Design review of the part built by this model. Coordinates are the model's own, in mm. A direction names the side the tool comes from. Coordinates: 2 decimals unless noted, no trailing zeros. Write each loop counter-clockwise with the first axis right and the second up, starting at its lowest first coordinate (ties: lowest second). Pieces come first, ordered by that corner, then holes. Notation, with made-up numbers: M -1.5,-11.75 L 31.5,-11.75 A20 cw 31.5,13.25 Z; hole C 12.5,-20 d8. An arc over 180 degrees is marked long. One line per question, with ' | ' between items.
from build123d import *

# Parameters (mm, degrees)
F1_DEPTH = 25
F3_DEPTH = 200
F5_DEPTH = 25


with BuildPart() as f1:
    # F0 (on Top) → F1 (new body)
    with BuildSketch(Plane.XY):
        Polygon((-401.6996773316, 377.6099345749), (-401.6996773316, -282.3900654251), (-151.6996773316, -282.3900654251), (258.3003226684, 127.6099345749), (258.3003226684, 377.6099345749), align=None)
    extrude(amount=F1_DEPTH)

    # F2 (on face) → F3 (join)
    with BuildSketch(Plane.XY.offset(25)):
        Polygon((-376.6996773316, -257.3900654251), (-376.6996773316, 352.6099345749), (233.3003226684, 352.6099345749), (233.3003226684, 127.6099345749), (258.3003226684, 127.6099345749), (258.3003226684, 377.6099345749), (-401.6996773316, 377.6099345749), (-401.6996773316, -282.3900654251), (-151.6996773316, -282.3900654251), (-151.6996773316, -257.3900654251), align=None)
    extrude(amount=F3_DEPTH)

    # F4 (on face) → F5 (join)
    with BuildSketch(Plane.XY.offset(225)):
        Polygon((-401.6996773316, -282.3900654251), (-151.6996773316, -282.3900654251), (-151.6996773316, -257.3900654251), (-376.6996773316, -257.3900654251), (-376.6996773316, 352.6099345749), (233.3003226684, 352.6099345749), (233.3003226684, 127.6099345749), (258.3003226684, 127.6099345749), (258.3003226684, 377.6099345749), (-401.6996773316, 377.6099345749), align=None)
        Polygon((-151.6996773316, -257.3900654251), (-151.6996773316, -282.3900654251), (258.3003226684, 127.6099345749), (233.3003226684, 127.6099345749), (233.3003226684, 352.6099345749), (-376.6996773316, 352.6099345749), (-376.6996773316, -257.3900654251), align=None)
    extrude(amount=F5_DEPTH)


solid = f1.part
1. Draft analysis for pull direction Z (two halves, no side actions). For faces 5 (the face through (-134, 110, 225)), 6 (the face through (-150, 126, 250)), 7 (the face through (-67, 377.61, 123)), state which applies: pulls with the +Z half, pulls with the -Z half, needs draft (parallel to the pull), parting line crosses it, or undercut.
Answer sheet:
face 5: undercut | face 6: pulls with the +Z half | face 7: needs draft
2. Take a section at C-C (z = 69.5). Write out the cut boundary in (x, y), then the cut area to 3 significant figures.
Answer sheet:
outline: M -401.7,-282.39 L -151.7,-282.39 L -151.7,-257.39 L -376.7,-257.39 L -376.7,352.61 L 233.3,352.61 L 233.3,127.61 L 258.3,127.61 L 258.3,377.61 L -401.7,377.61 Z | area: 43,600 mm^2
3. Tool access review of faces 1 (the face through (-134, 110, 25)), 2 (the face through (-151.7, -270, 124)), 3 (the face through (233.3, 242, 124)), 4 (the face through (-263, -257.39, 124)): name each direction out of +Z, -Z, +X, -X, +Y, -Y from which nothing blocks a thin tool from reaching the whole face with its end or side.
Answer sheet:
face 1: none | face 2: +X, -Y | face 3: -Y | face 4: +X
4. Take a section at D-D (x = 97.5). Write out the cut boundary in (y, z), then the cut area to 3 significant figures.
Answer sheet:
outline: M -33.19,0 L 377.61,0 L 377.61,250 L -33.19,250 L -33.19,225 L 352.61,225 L 352.61,25 L -33.19,25 Z | area: 25,500 mm^2
5. To check wall thickness, follow line 1 along Z through (x, y) = (-64.5, 11.5); line 2 along X through (y, z) = (230, 53); line 3 along Y through (x, z) = (-168, 44.5). State the ranges of each line that lie inside material, in increasing order. Write a range as [from, to].
Answer sheet:
line 1: [0, 25], [225, 250] | line 2: [-401.7, -376.7], [233.3, 258.3] | line 3: [-282.39, -257.39], [352.61, 377.61]
6. Take a section at A-A (x = -176). Write out the cut boundary in (y, z), then the cut area to 3 significant figures.
Answer sheet:
outline: M -282.39,0 L 377.61,0 L 377.61,250 L -282.39,250 Z; hole M -257.39,25 L 352.61,25 L 352.61,225 L -257.39,225 Z | area: 43,000 mm^2
7. Insertion check: pin 1 Ø4 at (x, y) = (-123.5, -134.5) entering from -Z; pin 2 Ø4 at (x, z) = (-4, 50) entering from -Y. Each pin has a flat end and moves straight along its axis. Give the tip position at first contact, or say it passes through.
Answer sheet:
pin 1: z = 0 | pin 2: y = 352.61
8. Take a section at B-B (y = 152). Write out the cut boundary in (x, z).
Answer sheet:
outline: M -401.7,0 L 258.3,0 L 258.3,250 L -401.7,250 Z; hole M -376.7,25 L 233.3,25 L 233.3,225 L -376.7,225 Z
